from build123d import *

# Parameters (mm, degrees)
SKETCH1_W           = 38.1
SKETCH1_H           = 4.7625
BOSS_EXTRUDE1_DEPTH = 127
SKETCH2_W           = 12.7
SKETCH2_H           = 6.35
BOSS_EXTRUDE2_DEPTH = 6.35
SKETCH3_R           = 1.499997
CUT_EXTRUDE1_DEPTH  = 138.389847924
FILLET1_R           = 2.54
SKETCH4_W           = 50.8
SKETCH4_H           = 38.1
CUT_EXTRUDE2_DEPTH  = 137.423436059
FILLET2_R           = 20.32
SKETCH5_R           = 4.445
CUT_EXTRUDE3_DEPTH  = 137.423436059
FILLET3_R           = 25.4


with BuildPart() as part:
    # Sketch1 → Boss-Extrude1 (new body)
    with BuildSketch(Plane(origin=(0, 0, 0), x_dir=(0, 0, -1), z_dir=(1, 0, 0))):
        Polygon((0, 30.1625), (0, 0), (-42.8625, 0), (-42.8625, 4.7625), (-4.7625, 4.7625), (-4.7625, 30.1625), align=None)
        with Locations((19.05, 2.38125)):
            Rectangle(SKETCH1_W, SKETCH1_H)
    extrude(amount=BOSS_EXTRUDE1_DEPTH)

    # Sketch2 → Boss-Extrude2 (add)
    with BuildSketch(Plane(origin=(0, 4.7625, 0), x_dir=(1, 0, 0), z_dir=(0, 1, 0))):
        with Locations((63.5, -20.6375)):
            Rectangle(SKETCH2_W, SKETCH2_H)
    extrude(amount=BOSS_EXTRUDE2_DEPTH)

    # Sketch3 → Cut-Extrude1 (cut, through all)
    with BuildSketch(Plane.XY.offset(4.7625)):
        with Locations((63.5, 23.8125)):
            Circle(SKETCH3_R)
    extrude(amount=-CUT_EXTRUDE1_DEPTH, mode=Mode.SUBTRACT)

    # Fillet1
    fillet1_edges = [part.edges().sort_by_distance(p)[0] for p in [
        (57.15, 11.1125, 20.6375),
        (63.5, 11.1125, 23.8125),
        (69.85, 11.1125, 20.6375),
        (63.5, 11.1125, 17.4625),
    ]]
    fillet(fillet1_edges, radius=FILLET1_R)

    # Sketch4 → Cut-Extrude2 (cut, through all)
    with BuildSketch(Plane(origin=(0, 4.7625, 0), x_dir=(1, 0, 0), z_dir=(0, 1, 0))):
        with Locations((63.5, 19.05)):
            Rectangle(SKETCH4_W, SKETCH4_H)
    extrude(amount=-CUT_EXTRUDE2_DEPTH, mode=Mode.SUBTRACT)

    # Fillet2
    # the kernel refuses this fillet: 20.32 mm, written as the material it takes off along each edge
    with BuildSketch(Plane(origin=(0, -50.8, -38.1), x_dir=(0, 0, 1), z_dir=(0, 1, 0)), Plane(origin=(88.9, 55.5625, -38.1), x_dir=(1, 0, 0), z_dir=(0, -1, 0))) as fillet2_piece_1:
        with BuildLine():
            CenterArc((FILLET2_R, FILLET2_R), FILLET2_R, 180, 90)
            Line((0, FILLET2_R), (0, 0))
            Line((0, 0), (FILLET2_R, 0))
        make_face()
    extrude(amount=106.3625, mode=Mode.SUBTRACT)
    with BuildSketch(Plane(origin=(38.1, 55.5625, -38.1), x_dir=(-1, 0, 0), z_dir=(0, -1, 0)), Plane(origin=(127, -50.8, -38.1), x_dir=(0, 0, 1), z_dir=(0, 1, 0))) as fillet2_piece_2:
        with BuildLine():
            CenterArc((FILLET2_R, -FILLET2_R), FILLET2_R, 90, 90)
            Line((0, -FILLET2_R), (0, 0))
            Line((0, 0), (FILLET2_R, 0))
        make_face()
    extrude(amount=106.3625, mode=Mode.SUBTRACT)

    # Sketch5 → Cut-Extrude3 (cut, through all)
    with BuildSketch(Plane(origin=(0, 4.7625, 0), x_dir=(1, 0, 0), z_dir=(0, 1, 0))):
        with Locations(Location((12.7, -13.6525, 0), (0, 0, 270))):
            Circle(SKETCH5_R)
        with Locations(Location((12.7, -33.9725, 0), (0, 0, 270))):
            Circle(SKETCH5_R)
        with Locations(Location((114.3, -13.6525, 0), (0, 0, 270))):
            Circle(SKETCH5_R)
        with Locations(Location((114.3, -33.9725, 0), (0, 0, 270))):
            Circle(SKETCH5_R)
        with Locations(Location((38.1, -13.6525, 0), (0, 0, 270))):
            Circle(SKETCH5_R)
        with Locations(Location((88.9, -13.6525, 0), (0, 0, 270))):
            Circle(SKETCH5_R)
        with Locations(Location((38.1, -33.9725, 0), (0, 0, 270))):
            Circle(SKETCH5_R)
        with Locations(Location((88.9, -33.9725, 0), (0, 0, 270))):
            Circle(SKETCH5_R)
    extrude(amount=-CUT_EXTRUDE3_DEPTH, mode=Mode.SUBTRACT)

    # Fillet3
    fillet3_edges = [part.edges().sort_by_distance(p)[0] for p in [
        (127, 30.1625, 2.38125),
        (0, 30.1625, 2.38125),
    ]]
    fillet(fillet3_edges, radius=FILLET3_R)


solid = part.part
The listing builds one solid part. Answer for the finished solid, in the listing's coordinates (mm). A direction names the side the tool comes from. Coordinates: 2 decimals unless noted, no trailing zeros. Order: outer loops, then holes, each group sorted by start corner. A loop starts at its lowest first (then second) coordinate and runs counter-clockwise, first axis right, second up.
Q1. A cutting plane is placed at B-B, the plane x = 63.5. Write down the section's boundary in (y, z), and give its area (3 significant figures).
Q2. For a pull along Z with two mould halves and no side action, classify faces 1 (the face through (41.85, 2.41, 16.04)), 2 (the face through (63.589, 10.349, 23.088)), 3 (the face through (7.24, 22.52, 2.35)) as pulls with the +Z half, pulls with the -Z half, needs draft (parallel to the pull), parting line crosses it, or undercut.
Q3. A cutting plane is placed at D-D, the plane y = 15. Write down the section's boundary in (x, z), and give its area (3 significant figures).
Q4. Which of the six approach directions +Z, -Z, +X, -X, +Y, -Y give full straight-line access (tool end or side, diameter ignored) to faces 4 (the face through (63, 7, 23.812)), 5 (the face through (69.407, 10.006, 20.593)), 6 (the face through (108, 4.762, -19))?
Q5. Given P1, Ø6, axis at y = 20.5, z = 3, coming from the -X side; P2, Ø10, axis at x = 12.7, z = 13.65, coming from the +Y side; P3, Ø4, axis at x = 20.5, y = 20, coming from the -Z side, each flat-ended and moving along its own axis, determine where each tip first touches the part or whether it passes through.
Q6. A cutting plane is placed at A-A, the plane y = 3. State how many separate pieces and enclosed holes the cut face has, and give its area (3 significant figures).
Q7. Consider line 1 (X direction, y = 4, z = -8.5); line 2 (Z direction, x = 36, y = 6). Determine where each line is inside the solid, lowest interval first.
Q8. A cutting plane is placed at C-C, the plane x = 12.7. Write down the section's boundary in (y, z), and give its area (3 significant figures).
Answers follow:
1. outline: (0, 0) - (22.31, 0) - (22.31, 4.76) - (4.76, 4.76) - (4.76, 17.46) - (8.57, 17.46) arc R2.54 ccw to (11.11, 20) - (11.11, 21.27) arc R2.54 ccw to (8.57, 23.81) - (4.76, 23.81) - (4.76, 42.86) - (0, 42.86) - close; (25.31, 0) - (30.16, 0) - (30.16, 4.76) - (25.31, 4.76) - close
1. area: 348 mm2
2. face 1: undercut
2. face 2: pulls with the +Z half
2. face 3: needs draft
3. outline: (2.15, 0) - (124.85, 0) - (124.85, 4.76) - (2.15, 4.76) - close
3. area: 584 mm2
4. face 4: +Z, +X, -X, +Y
4. face 5: +Z, +X, +Y
4. face 6: -Z, +X, -X, +Y
5. P1: stops at x = 3.42
5. P2: stops at y = 4.76
5. P3: stops at z = 0
6. separate pieces: 1
6. enclosed holes: 8
6. area: 7,500 mm2
7. line 1: x = 0 to 38.1, 88.9 to 127
7. line 2: z = 0 to 4.76
8. outline: (0, -36.62) - (4.76, -36.62) - (4.76, 0) - (26.76, 0) - (26.76, 4.76) - (4.76, 4.76) - (4.76, 9.21) - (0, 9.21) - close; (0, 18.1) - (4.76, 18.1) - (4.76, 29.53) - (0, 29.53) - close; (0, 38.42) - (4.76, 38.42) - (4.76, 42.86) - (0, 42.86) - close
8. area: 399 mm2
